Verification items for the finished model (mm, model axes). Face numbers are marked on the shaded views. Give positions to 0.01 mm unless a question says otherwise; leave off trailing zeros. Order: outer loops, then holes, each group sorted by start corner. A loop starts at its lowest first (then second) coordinate and runs counter-clockwise, first axis right, second up. Notation, with made-up numbers: M 60,73.25 L 74,73.25 A21 ccw 74,109.25 Z; hole C -7.5,-29.75 d5. An arc over 180 degrees is marked long. Answer as a JSON object with one key per item and string values.
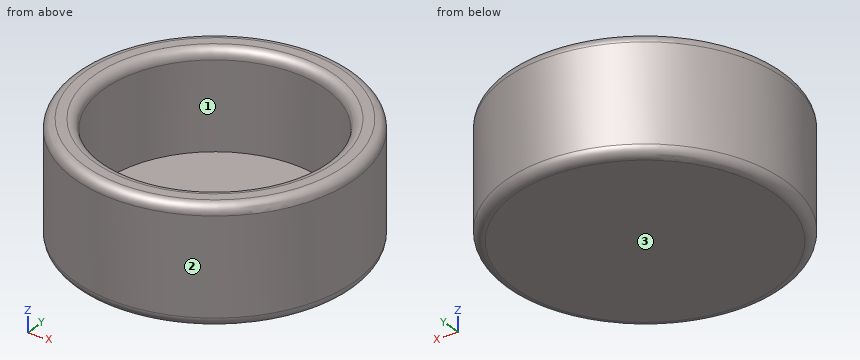
```python
from build123d import *

# Parameters (mm, degrees)
F0_R     = 14.5
F0_R_2   = 11.5
F1_DEPTH = 10
F2_R     = 14.5
F3_DEPTH = 2
F4_R     = 1


with BuildPart() as f1:
    # F0 (on Top) → F1 (new body)
    with BuildSketch(Plane.XY):
        Circle(F0_R)
        Circle(F0_R_2, mode=Mode.SUBTRACT)
    extrude(amount=F1_DEPTH)

    # F2 (on face) → F3 (join)
    with BuildSketch(Plane(origin=(0, 0, 0), x_dir=(1, 0, 0), z_dir=(0, 0, -1))):
        Circle(F2_R)
    extrude(amount=F3_DEPTH)

    # F4
    f4_edges = [f1.edges().sort_by_distance(p)[0] for p in [
        (-14.5, 0, 10),
        (-11.5, 0, 10),
        (-14.5, 0, -2),
    ]]
    fillet(f4_edges, radius=F4_R)


solid = f1.part
```
Q1. Material ranges on L1, parallel to Y at x = 0, z = 4.5; L2, parallel to Z at x = -3.75, y = 1; L3, parallel to X at y = 3.75, z = 2.25, recorded low to high.
Resolved:
{"L1": "y = -14.5 to -11.5, 11.5 to 14.5", "L2": "z = -2 to 0", "L3": "x = -14.01 to -10.87, 10.87 to 14.01"}
Q2. Section check A-A on y = 0. Record the cut outline in (x, z), then the cut area to 3 significant figures.
Resolved:
{"outline": "M -14.5,-1 A1 ccw -13.5,-2 L 13.5,-2 A1 ccw 14.5,-1 L 14.5,9 A1 ccw 13.5,10 L 12.5,10 A1 ccw 11.5,9 L 11.5,0 L -11.5,0 L -11.5,9 A1 ccw -12.5,10 L -13.5,10 A1 ccw -14.5,9 Z", "area": "117 mm²"}
Q3. Release check for a two-part mould opening along X. For the marked faces 1, 2 and 3 record: +X half, -X half, draft (parallel to the pull), parting line (faces both ways), or undercut.
Resolved:
{"face 1": "undercut", "face 2": "parting line", "face 3": "draft"}
Q4. Section check C-C on z = 7.5. Record the cut outline in (x, y).
Resolved:
{"outline": "C 0,0 d29; hole C 0,0 d23"}
Q5. Gauge pin test, flat ends, axial feed: pin 1 Ø3 at (x, z) = (-0.5, 0) entering from +Y; pin 2 Ø4 at (y, z) = (9, 1.5) entering from -X; pin 3 Ø2 at (x, z) = (7, 3.5) entering from +Y; pin 4 Ø1.5 at (x, y) = (-1, -11) entering from +Z. Record the tip position at first contact, or that the pin passes through.
Resolved:
{"pin 1": "stops at y = 14.5", "pin 2": "stops at x = -12.7", "pin 3": "stops at y = 13.2", "pin 4": "stops at z = 9.71"}
